Verification items for the finished model (mm, model axes). A direction names the side the tool comes from. Give positions to 0.01 mm unless a question says otherwise; leave off trailing zeros. Write each loop counter-clockwise with the first axis right and the second up, starting at its lowest first coordinate (ties: lowest second). Pieces come first, ordered by that corner, then holes. Notation, with made-up numbers: (68, -16.75) -> (82, -16.75) arc R29 cw to (82, 16.25) -> close; hole circle Ø1 at (79, 13). An arc over 180 degrees is marked (long way). Answer as CSV lines item,"result". Start each with the question number.
1) Sectioned sample at B-B on y = -1.5. Record the cut outline in (x, z) (3 decimals).
2) Material ranges on L1, parallel to X at y = -3.75, z = 2.5 (3 decimals); L2, parallel to Z at x = 0.25, y = -19.25; L3, parallel to X at y = -2.75, z = 6.5 (3 decimals), recorded low to high.
3) Sectioned sample at C-C on z = 3.25. Record the cut outline in (x, y) (3 decimals).
4) Tool access check on faces 1 (the flat face through (7, -9.525, 7)), 2 (the flat face through (6.35, -10, 0)), 3 (the flat face through (7, -9.525, -7)), 4 (the flat face through (-7, -9.525, 7)). Record the directions out of +Z, -Z, +X, -X, +Y, -Y that give a thin tool (end or side, any length) a straight path to the whole face; none if there is none.
5) Sectioned sample at A-A on x = -2. Record the cut outline in (y, z) (3 decimals).
6) Mould release check, pull along X, two halves, no side actions. Record for faces 5 (the flat face through (9.525, -5, 0)), 6 (the flat face through (-3.219, -10.018, -5.474)), 7 (the cylindrical face through (-8.417, -4.696, -8.45)): released by +X, released by -X, zero draft, split by the parting line, or undercut.
7) Sectioned sample at D-D on x = 7.5. Record the cut outline in (y, z) (3 decimals).
8) Gauge pin test, flat ends, axial feed: pin 1 Ø1 at (x, z) = (-4, 2) entering from +Y; pin 2 Ø2 at (x, z) = (0.5, -6.5) entering from -Y; pin 3 Ø2 at (y, z) = (-15, 3) entering from +X; pin 4 Ø2 at (x, y) = (-2.5, -16.5) entering from -Z. Record the tip position at first contact, or that the pin passes through.
Autodesk Inventor part; units mm, degrees
ref_plane "YZ Plane" through (0, 0, 0) normal (1, 0, 0) x (0, 1, 0)
ref_plane "XZ Plane" through (0, 0, 0) normal (0, 1, 0) x (-1, 0, 0)
ref_plane "XY Plane" through (0, 0, 0) normal (0, 0, 1) x (1, 0, 0)
sketch "Sketch1" plane through (0, 0, 0) normal (0, 1, 0) x (-1, 0, 0)
  line L0 (6.35, -3.6662) -> (0, -7.3323)
  line L1 (0, -7.3323) -> (-6.35, -3.6662)
  line L2 (-6.35, -3.6662) -> (-6.35, 3.6662)
  line L3 (-6.35, 3.6662) -> (0, 7.3323)
  line L4 (0, 7.3323) -> (6.35, 3.6662)
  line L5 (6.35, 3.6662) -> (6.35, -3.6662)
  line L6 (9.525, 7.1772) -> (9.525, -7.1772)
  line L7 (-9.525, 7.1772) -> (-9.525, -7.1772)
  line L8 (7.1772, 9.525) -> (-7.1772, 9.525)
  line L9 (7.1772, -9.525) -> (-7.1772, -9.525)
  arc A0 (7.1772, -9.525) -> (9.525, -7.1772) centre (0, 0) ccw
  arc A1 (9.525, 7.1772) -> (7.1772, 9.525) centre (0, 0) ccw
  arc A2 (-7.1772, 9.525) -> (-9.525, 7.1772) centre (0, 0) ccw
  arc A3 (-9.525, -7.1772) -> (-7.1772, -9.525) centre (0, 0) ccw
  dimension "d0" = 12.7
  dimension "d9" = 9.525
  dimension "d10" = 9.525
  dimension "d11" = 9.525
  dimension "d12" = 9.525
extrude "Extrusion1" add sketch "Sketch1" against normal blind 9.525 contours L0 L1 L2 L3 L4 L5 | L6 A0 L9 A3 L7 A2 L8 A1
sketch "Sketch2" plane through (0, -9.525, 0) normal (0, -1, 0) x (0.7071, 0, 0.7071)
  circle A0 centre (0, 0) radius 9.525
  dimension "d4" = 19.05
extrude "Extrusion2" add sketch "Sketch2" along normal blind 10.795
extrude "Extrusion3" cut sketch "Sketch1" against normal through all contours L0 L1 L2 L3 L4 L5
properties part number "T81H-RS81" material "Aluminum 6061"
Ans:
1,outline,"(-9.525, -7.177) arc R11.926 ccw to (-7.177, -9.525) -> (7.177, -9.525) arc R11.926 ccw to (9.525, -7.177) -> (9.525, 7.177) arc R11.926 ccw to (7.177, 9.525) -> (-7.177, 9.525) arc R11.926 ccw to (-9.525, 7.177) -> close; hole (-6.35, -3.666) -> (0, -7.332) -> (6.35, -3.666) -> (6.35, 3.666) -> (0, 7.332) -> (-6.35, 3.666) -> close"
2,L1,"x = -9.525 to -6.35, 6.35 to 9.525"
2,L2,"z = -9.52 to -7.19, 7.19 to 9.52"
2,L3,"x = -9.525 to -1.442, 1.442 to 9.525"
3,outline,"(-9.525, -9.525) -> (-8.953, -9.525) -> (-8.953, -20.32) -> (-6.35, -20.32) -> (-6.35, 0) -> (-9.525, 0) -> close; (6.35, -20.32) -> (8.953, -20.32) -> (8.953, -9.525) -> (9.525, -9.525) -> (9.525, 0) -> (6.35, 0) -> close"
4,face 1,"+Z, +X, -Y"
4,face 2,"+Y, -Y"
4,face 3,"-Z, +X, -Y"
4,face 4,"+Z, -X, -Y"
5,outline,"(-20.32, -9.313) -> (-9.525, -9.313) -> (-9.525, -9.525) -> (0, -9.525) -> (0, -6.178) -> (-20.32, -6.178) -> close; (-20.32, 6.178) -> (0, 6.178) -> (0, 9.525) -> (-9.525, 9.525) -> (-9.525, 9.313) -> (-20.32, 9.313) -> close"
6,face 5,"released by +X"
6,face 6,"undercut"
6,face 7,"released by -X"
7,outline,"(-20.32, -5.872) -> (-9.525, -5.872) -> (-9.525, -9.273) -> (0, -9.273) -> (0, 9.273) -> (-9.525, 9.273) -> (-9.525, 5.872) -> (-20.32, 5.872) -> close"
8,pin 1,"passes through"
8,pin 2,"stops at y = -20.32"
8,pin 3,"stops at x = 9.31"
8,pin 4,"stops at z = -9.41"
